The listing builds one solid part. Answer for the finished solid, in the listing's coordinates (mm). Face numbers are marked on the shaded views. A direction names the side the tool comes from. Round coordinates to 2 decimals unless told otherwise and drop trailing zeros. Write each loop counter-clockwise with the first axis right and the second up, starting at its lowest first coordinate (ties: lowest second). Pieces come first, ordered by that corner, then holes.
Item 1: Find section B-B on z = -8.89. Give the vertices of the cut face in (x, y) (3 decimals).
Item 2: Find section A-A on z = 5.5. Give the vertices of the cut face in (x, y) (3 decimals), then the cut area to 3 significant figures.
Item 3: This flat-tipped pin is pushed along its axis until it touches: pin 1 (1.5 mm diameter, centred on y = -1.5, z = -9.5, fed in from +X). Where does it stop, or does it pass through?
Item 4: Find section D-D on y = -1.65. Give the number of separate pieces and of enclosed holes in the cut face, then the cut area to 3 significant figures.
Item 5: Find the intervals of material crossed by probe 1 along X at (y, z) = (-0.5, -7.5); probe 2 along X at (y, z) = (-3, 6); probe 3 along Z at (x, y) = (-5.25, -2.85), in increasing order.
Item 6: A tool of negligible diameter and unlimited length cuts with its end or side. For the marked faces 1, 2, 3, 4 and 5, from which of +Z, -Z, +X, -X, +Y, -Y can it reach the whole face along a straight path? Write none if from no direction.
Item 7: For a pull along X with two mould halves and no side action, classify the marked faces 6, 7 and 8 as +X half, -X half, draft (parallel to the pull), parting line (faces both ways), or undercut.
Item 8: Find section C-C on x = -8.89. Give the vertices of the cut face in (y, z) (3 decimals), then the cut area to 3 significant figures.
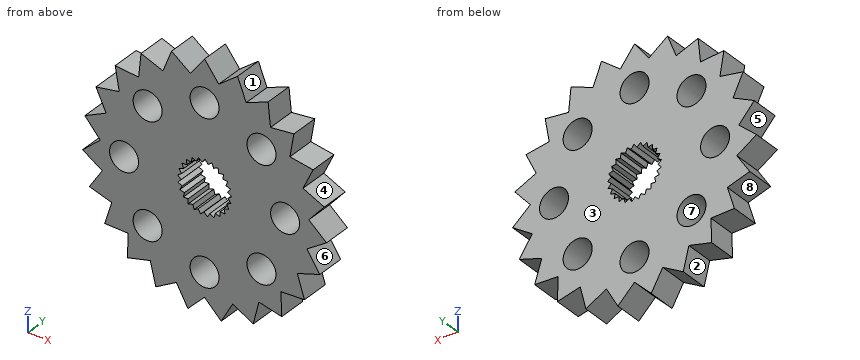
```python
from build123d import *

# Parameters (mm, degrees)
F0_R     = 1.6
F1_DEPTH = 3.175


with BuildPart() as f1:
    # F0 (on Front) → F1 (new body)
    with BuildSketch(Plane.XZ):
        Polygon((1.570599, 11.426958), (0, 13.5), (-1.570599, 11.426958), (-3.642256, 12.999383), (-4.595314, 10.579473), (-7.014383, 11.534662), (-7.279214, 8.947356), (-9.866286, 9.214467), (-9.423249, 6.651656), (-11.98645, 6.210878), (-10.868405, 3.862632), (-13.217635, 2.746656), (-11.507501, 0.787135), (-13.468528, -0.921273), (-11.293138, -2.346741), (-12.720522, -4.520875), (-10.241214, -5.30657), (-11.029094, -7.785184), (-8.429747, -7.872834), (-8.519687, -10.472102), (-5.993084, -9.855207), (-5.378415, -12.382353), (-3.111941, -11.106663), (-1.83825, -13.37426), (0, -11.53439), (1.83825, -13.37426), (3.111941, -11.106663), (5.378415, -12.382353), (5.993084, -9.855207), (8.519687, -10.472102), (8.429747, -7.872834), (11.029094, -7.785184), (10.241214, -5.30657), (12.720522, -4.520875), (11.293138, -2.346741), (13.468528, -0.921273), (11.507501, 0.787135), (13.217635, 2.746656), (10.868405, 3.862632), (11.98645, 6.210878), (9.423249, 6.651656), (9.866286, 9.214467), (7.279214, 8.947356), (7.014383, 11.534662), (4.595314, 10.579473), (3.642256, 12.999383), align=None)
        with Locations((-8.89, 0)):
            Circle(F0_R, mode=Mode.SUBTRACT)
        with Locations((-6.286179, -6.286179)):
            Circle(F0_R, mode=Mode.SUBTRACT)
        with Locations((0, -8.89)):
            Circle(F0_R, mode=Mode.SUBTRACT)
        with Locations((6.286179, -6.286179)):
            Circle(F0_R, mode=Mode.SUBTRACT)
        Polygon((-2.313127, 1.150841), (-2.481189, 1.651718), (-1.954254, 1.689937), (-1.992473, 2.216873), (-1.472587, 2.122848), (-1.378562, 2.642733), (-0.898392, 2.422372), (-0.678031, 2.902541), (-0.267748, 2.56969), (0.065104, 2.979972), (0.37972, 2.555544), (0.804147, 2.87016), (1.003328, 2.380825), (1.492663, 2.580005), (1.563894, 2.056509), (2.08739, 2.12774), (2.026194, 1.602976), (2.550958, 1.54178), (2.361181, 1.048721), (2.85424, 0.858945), (2.547807, 0.428572), (2.97818, 0.122139), (2.574344, -0.218506), (2.914989, -0.622342), (2.439126, -0.851855), (2.668639, -1.327718), (2.150649, -1.431678), (2.254609, -1.949669), (1.727038, -1.921544), (1.698914, -2.449115), (1.194912, -2.290672), (1.036469, -2.794674), (0.587704, -2.515869), (0.308899, -2.964634), (-0.056431, -2.582985), (-0.43808, -2.948314), (-0.69702, -2.487802), (-1.157533, -2.746742), (-1.293813, -2.236301), (-1.804254, -2.372581), (-1.809311, -1.844285), (-2.337607, -1.849342), (-2.211123, -1.336386), (-2.724079, -1.209903), (-2.474002, -0.744517), (-2.939388, -0.494441), (-2.581431, -0.105868), (-2.970004, 0.252089), (-2.526659, 0.539434), (-2.814004, 0.982779), align=None, mode=Mode.SUBTRACT)
        with Locations((8.89, 0)):
            Circle(F0_R, mode=Mode.SUBTRACT)
        with Locations((-6.286179, 6.286179)):
            Circle(F0_R, mode=Mode.SUBTRACT)
        with Locations((6.286179, 6.286179)):
            Circle(F0_R, mode=Mode.SUBTRACT)
        with Locations((0, 8.89)):
            Circle(F0_R, mode=Mode.SUBTRACT)
    extrude(amount=F1_DEPTH)


solid = f1.part
```
Check values:
1. outline: (-8.465, -3.175) - (-1.6, -3.175) - (-1.6, 0) - (-8.465, 0) - close; (1.6, -3.175) - (8.465, -3.175) - (8.465, 0) - (1.6, 0) - close
2. outline: (-11.648, -3.175) - (-7.68, -3.175) - (-7.68, 0) - (-11.648, 0) - close; (-4.893, -3.175) - (4.893, -3.175) - (4.893, 0) - (-4.893, 0) - close; (7.68, -3.175) - (11.648, -3.175) - (11.648, 0) - (7.68, 0) - close
2. area: 56.3 mm2
3. pin 1: stops at x = 8.51
4. separate pieces: 1
4. enclosed holes: 9
4. area: 399 mm2
5. probe 1: x = -10.94 to -7.33, -5.24 to -0.79, 0.79 to 5.24, 7.33 to 10.94
5. probe 2: x = -11.89 to -7.86, -4.71 to 4.71, 7.86 to 11.89
5. probe 3: z = -12.31 to -7.51, -5.07 to 5.07, 7.51 to 10.84
6. face 1: +Z, +Y, -Y
6. face 2: -Z, +Y, -Y
6. face 3: +Z, -Z, +X, -X, +Y
6. face 4: +X, +Y, -Y
6. face 5: -X, +Y, -Y
7. face 6: +X half
7. face 7: undercut
7. face 8: -X half
8. outline: (-3.175, -7.857) - (0, -7.857) - (0, -1.6) - (-3.175, -1.6) - close; (-3.175, 1.6) - (0, 1.6) - (0, 9.114) - (-3.175, 9.114) - close
8. area: 43.7 mm2
